```python
from build123d import *

# Parameters (mm, degrees)
F3_W     = 3
F3_H     = 0.4
F4_DEPTH = 1


with BuildPart() as f1:
    # F0 (on Front) → F1 (revolve)
    with BuildSketch(Plane.XZ):
        with BuildLine():
            Line((0, 9.5), (0, 0))
            Line((0, 0), (0.75, 0.75))
            Line((0.75, 0.75), (0.75, 8))
            Line((0.75, 8), (1.5, 8))
            ThreePointArc((1.5, 8), (1.06066, 9.06066), (0, 9.5))
        make_face()
    revolve(axis=Axis((0, 0, 4.75), (0, 0, 1)))

    # F3 (on offset) → F4 (cut)
    with BuildSketch(Plane.XY.offset(9.5)):
        Rectangle(F3_W, F3_H)
    extrude(amount=-F4_DEPTH, mode=Mode.SUBTRACT)


solid = f1.part
```
Work out the finished part from the listing and answer in its coordinate system (mm). A direction names the side the tool comes from. Coordinates: 2 decimals unless noted, no trailing zeros. Write each loop counter-clockwise with the first axis right and the second up, starting at its lowest first coordinate (ties: lowest second). Pieces come first, ordered by that corner, then holes.
Q1. Which of the six approach directions +Z, -Z, +X, -X, +Y, -Y give full straight-line access (tool end or side, diameter ignored) to faces 1 (the face through (0, 0, 0)), 2 (the face through (0, 0.2, 9))?
Q2. Find the intervals of material crossed by line 1 (X direction, y = -1.2, z = 8.5); line 2 (Z direction, x = -0.5, y = 0.75), in increasing order.
Q3. Determine the mould class of faces 3 (the face through (0, 1, 8)), 4 (the face through (-0.75, 0.03, 4.43)), 5 (the face through (0, -0.2, 9)) for opening direction Y: released by +Y, released by -Y, zero draft, split by the parting line, or undercut.
Q4. A cutting plane is placed at A-A, the plane z = 3. Give the vertices of the cut face in (x, y).
Q5. Each of these flat-tipped pins is pushed along its axis until it touches: pin 1 Ø0.5 at (x, z) = (0.5, 9) entering from -Y; pin 2 Ø1.5 at (y, z) = (0.5, 4.5) entering from +X; pin 3 Ø1.5 at (x, y) = (0.5, 0.5) entering from -Z. Where does it stop, or does it pass through?
Findings below:
1. face 1: -Z
1. face 2: +Z, +X, -X
2. line 1: x = -0.75 to 0.75
2. line 2: z = 8 to 9.2
3. face 3: zero draft
3. face 4: split by the parting line
3. face 5: undercut
4. outline: circle Ø1.5 at (0, 0)
5. pin 1: stops at y = -1.22
5. pin 2: stops at x = 0.75
5. pin 3: stops at z = 0
